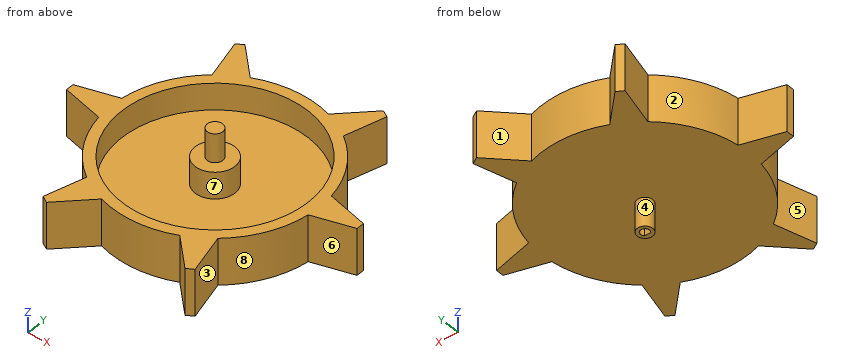
from build123d import *

# Parameters (mm, degrees)
SKETCH1_R                = 39
BOSS_EXTRUDE1_DEPTH      = 17.5
BOSS_EXTRUDE5_DEPTH      = 10.75
BOSS_EXTRUDE5_DEPTH_BACK = 28.25
SKETCH3_R                = 2.95
CUT_EXTRUDE1_START       = 10.75
CUT_EXTRUDE1_DEPTH       = 7.5
CIRPATTERN1_COUNT        = 6
SKETCH4_R                = 35
SKETCH4_R_2              = 7.5
CUT_EXTRUDE2_DEPTH       = 10


with BuildPart() as part:
    # Sketch1 → Boss-Extrude1 (new body)
    with BuildSketch(Plane.XY):
        Circle(SKETCH1_R)
        with BuildLine():
            Line((-54, 0), (-54, -3))
            Line((-54, -3), (-38.329847519, -7.198804702))
            ThreePointArc((-38.329847519, -7.198804702), (-38.968072448, -1.577760972), (-38.786367534, 4.076480533))
            Line((-38.786367534, 4.076480533), (-54, 0))
        make_face()
        with BuildLine():
            ThreePointArc((-38.786367534, 4.076480533), (-38.968072448, -1.577760972), (-38.329847519, -7.198804702))
            ThreePointArc((-38.329847519, -7.198804702), (3.614965197, -38.832100466), (39, 0))
            ThreePointArc((39, 0), (2.041037259, 38.946555264), (-38.786367534, 4.076480533))
        make_face()
    boss_extrude1 = extrude(amount=BOSS_EXTRUDE1_DEPTH)

    # Sketch3 → Boss-Extrude5 (add, two sides: drawn at the far end of the back side and taken through both)
    with BuildSketch(Plane.XY.offset(17.5).offset(-BOSS_EXTRUDE5_DEPTH_BACK)):
        Circle(SKETCH3_R)
    extrude(amount=BOSS_EXTRUDE5_DEPTH + BOSS_EXTRUDE5_DEPTH_BACK)

    # Sketch2 → Cut-Extrude1 (cut)
    with BuildSketch(Plane(origin=(0, 0, 0), x_dir=(-1, 0, 0), z_dir=(0, 0, -1)).offset(CUT_EXTRUDE1_START)):
        with BuildLine():
            Line((-1.223764683, -1.18), (1.223764683, -1.18))
            ThreePointArc((1.223764683, -1.18), (0, 1.7), (-1.223764683, -1.18))
        make_face()
    extrude(amount=-CUT_EXTRUDE1_DEPTH, mode=Mode.SUBTRACT)

    # CirPattern1: Boss-Extrude1 ×6 about axis
    cirpattern1_axis = Axis((0, 0, 0), (0, 0, 1))
    for i in range(1, CIRPATTERN1_COUNT):
        add(boss_extrude1.rotate(cirpattern1_axis, i * 360 / CIRPATTERN1_COUNT))

    # Sketch4 → Cut-Extrude2 (cut)
    with BuildSketch(Plane.XY.offset(17.5)):
        Circle(SKETCH4_R)
        Circle(SKETCH4_R_2, mode=Mode.SUBTRACT)
    extrude(amount=-CUT_EXTRUDE2_DEPTH, mode=Mode.SUBTRACT)


solid = part.part
Can you work these out from the model? Positions are in its coordinate system, mm. Face numbers are marked on the shaded views. A direction names the side the tool comes from. Coordinates: 2 decimals unless noted, no trailing zeros. Write each loop counter-clockwise with the first axis right and the second up, starting at its lowest first coordinate (ties: lowest second). Pieces come first, ordered by that corner, then holes. Notation, with made-up numbers: (-27.5, 84) - (2.5, 84) arc R24 cw to (2.5, 105) - close; hole circle Ø1 at (56, -35.5). An arc over 180 degrees is marked (long way). Return JSON: item names as keys, results as strings. Group by question number.
Item 1: If we section it at D-D (z = -6): Write out the boundary of the cut face in (x, y), then the cut area to 3 significant figures.
Item 2: Please list where these lines run through material, in increasing order: probe 1 along Y at (x, z) = (0, 12); probe 2 along X at (y, z) = (0, -9); probe 3 along Z at (x, y) = (26, 26).
Item 3: If we section it at B-B (x = 0): Write out the boundary of the cut face in (y, z), then the cut area to 3 significant figures.
Item 4: If we section it at A-A (z = 10.5): Write out the boundary of the cut face in (x, y).
Item 5: If we section it at C-C (z = 25): Write out the boundary of the cut face in (x, y).
Item 6: Which directions (+Z, -Z, +X, -X, +Y, -Y) give clear straight access to the entire face, cutting with the end or side of a thin tool? Please do the marked faces 5, 6, 7 and 8.
Item 7: I'm going to push flat-ended pins straight in: pin 1 Ø2 at (x, y) = (26.5, -17.5) entering from +Z; pin 2 Ø2 at (x, z) = (0, -8) entering from +Y; pin 3 Ø10 at (x, y) = (-12.5, 35.5) entering from -Z. Where does each tip first touch, or does it pass through?
Item 8: We'd pull the mould along X, two halves only. Please class the marked faces 1, 2, 3 and 4: pulls with the +X half, pulls with the -X half, needs draft (parallel to the pull), parting line crosses it, or undercut.
Return value:
{
 "1": {"outline": "circle Ø5.9 at (0, 0); hole (-1.22, -1.18) - (1.22, -1.18) arc R1.7 ccw (long way) to start", "area": "19.1 mm^2"},
 "2": {"probe 1": "y = -39 to -35, -7.5 to 7.5, 35 to 39", "probe 2": "x = -2.95 to -1.7, 1.7 to 2.95", "probe 3": "z = 0 to 17.5"},
 "3": {"outline": "(-39, 0) - (-2.95, 0) - (-2.95, -10.75) - (-1.18, -10.75) - (-1.18, -3.25) - (1.7, -3.25) - (1.7, -10.75) - (2.95, -10.75) - (2.95, 0) - (39, 0) - (39, 17.5) - (35, 17.5) - (35, 7.5) - (7.5, 7.5) - (7.5, 17.5) - (2.95, 17.5) - (2.95, 28.25) - (-2.95, 28.25) - (-2.95, 17.5) - (-7.5, 17.5) - (-7.5, 7.5) - (-35, 7.5) - (-35, 17.5) - (-39, 17.5) - close", "area": "920 mm^2"},
 "4": {"outline": "(-54, -3) - (-38.33, -7.2) arc R39 ccw to (-22.92, -31.55) - (-27, -46.77) - (-24.4, -48.27) - (-12.93, -36.79) arc R39 ccw to (15.86, -35.63) - (27, -46.77) - (29.6, -45.27) - (25.4, -29.6) arc R39 ccw to (38.79, -4.08) - (54, 0) - (54, 3) - (38.33, 7.2) arc R39 ccw to (22.92, 31.55) - (27, 46.77) - (24.4, 48.27) - (12.93, 36.79) arc R39 ccw to (-15.86, 35.63) - (-27, 46.77) - (-29.6, 45.27) - (-25.4, 29.6) arc R39 ccw to (-38.79, 4.08) - (-54, 0) - close; circle Ø15 at (0, 0); hole circle Ø70 at (0, 0)"},
 "5": {"outline": "circle Ø5.9 at (0, 0)"},
 "6": {"face 5": "+Z, -Z, -X", "face 6": "+Z, -Z, +X, -Y", "face 7": "+Z", "face 8": "+Z, -Z, +X"},
 "7": {"pin 1": "stops at z = 7.5", "pin 2": "stops at y = 2.95", "pin 3": "stops at z = 0"},
 "8": {"face 1": "undercut", "face 2": "pulls with the -X half", "face 3": "pulls with the +X half", "face 4": "parting line crosses it"}
}
